from build123d import *

# Parameters (mm, degrees)
SKETCH1_W           = 60
SKETCH1_H           = 60
BOSS_EXTRUDE1_DEPTH = 6
BOSS_EXTRUDE2_DEPTH = 20


with BuildPart() as part:
    # Sketch1 → Boss-Extrude1 (new body)
    with BuildSketch(Plane(origin=(0, 0, 0), x_dir=(1, 0, 0), z_dir=(0, 1, 0))):
        Rectangle(SKETCH1_W, SKETCH1_H)
    extrude(amount=BOSS_EXTRUDE1_DEPTH)

    # Sketch2 → Boss-Extrude2 (add)
    with BuildSketch(Plane(origin=(0, 0, 0), x_dir=(1, 0, 0), z_dir=(0, 1, 0))):
        Polygon((-30, 30), (-30, -30), (-25, -30), (-25, 25), (30, 25), (30, 30), align=None)
    extrude(amount=-BOSS_EXTRUDE2_DEPTH)


solid = part.part
Can you work these out from the model? Positions are in its coordinate system, mm. A direction names the side the tool comes from. Round coordinates to 2 decimals unless told otherwise and drop trailing zeros. Order: outer loops, then holes, each group sorted by start corner. A loop starts at its lowest first (then second) coordinate and runs counter-clockwise, first axis right, second up. Notation, with made-up numbers: (24, 19.25) - (39, 19.25) arc R21 cw to (39, 23.25) - close; hole circle Ø1 at (79, 54.25). An arc over 180 degrees is marked (long way). Answer in a Markdown table with one row per item.
(1) For P1, Ø10, axis at y = -9, z = -2, coming from the +X side; P2, Ø1, axis at x = -0.5, y = -12, coming from the +Z side; P3, Ø12, axis at y = -14.5, z = -20.5, coming from the +X side, each with a flat end and sliding along its axis, tell me the tip position at first contact or that it passes through.
From the geometry:
| item | result |
|---|---|
| P1 | stops at x = -25 |
| P2 | stops at z = -25 |
| P3 | stops at x = 30 |
(2) Which directions (+Z, -Z, +X, -X, +Y, -Y) give clear straight access to the entire face, cutting with the end or side of a thin tool? Please do faces 1 (the face through (-7, 1, 30)), 2 (the face through (2, 0, 2)).
From the geometry:
| item | result |
|---|---|
| face 1 | +Z, +X, -X, +Y, -Y |
| face 2 | +Z, +X, -Y |
(3) Suppose I cut it at A-A, the plane z = -20.5. Please give me the cut outline in (x, y).
From the geometry:
| item | result |
|---|---|
| outline | (-30, -20) - (-25, -20) - (-25, 0) - (30, 0) - (30, 6) - (-30, 6) - close |
(4) Please list where these lines run through material, in increasing order: L1, parallel to Y at x = 1, z = -9.5; L2, parallel to Z at x = -21, y = -3.5. Write a range as from..to.
From the geometry:
| item | result |
|---|---|
| L1 | y = 0..6 |
| L2 | z = -30..-25 |
(5) Suppose I cut it at B-B, the plane y = -17. Please give me the cut outline in (x, z), plus the area to 3 significant figures.
From the geometry:
| item | result |
|---|---|
| outline | (-30, -30) - (30, -30) - (30, -25) - (-25, -25) - (-25, 30) - (-30, 30) - close |
| area | 575 mm2 |
